Design review of the part built by this model. Coordinates are the model's own, in mm. Coordinates: 2 decimals unless noted, no trailing zeros. Write each loop counter-clockwise with the first axis right and the second up, starting at its lowest first coordinate (ties: lowest second). Pieces come first, ordered by that corner, then holes.
Q1. Clearance check with a flat-ended pin moving along its axis: pin 1 Ø5 at (x, y) = (-40.5, -4.5) entering from -Z. State where the tip first meets the part, or that it passes through.
Q2. Add section D-D, the plane y = -43. Give the boundary of the cut face in (x, z).
Q3. To check wall thickness, follow probe 1 along Y at (x, z) = (0, 0.85); probe 2 along Y at (x, z) = (17.5, 1.75); probe 3 along X at (y, z) = (0, 1.35). State the ranges of each line that lie inside material, in increasing order.
Q4. Add section C-C, the plane x = 0. Give the boundary of the cut face in (y, z).
Q5. Add section B-B, the plane z = 2.1. Give the boundary of the cut face in (x, y).
Q6. Add section A-A, the plane y = -14. Give the boundary of the cut face in (x, z).
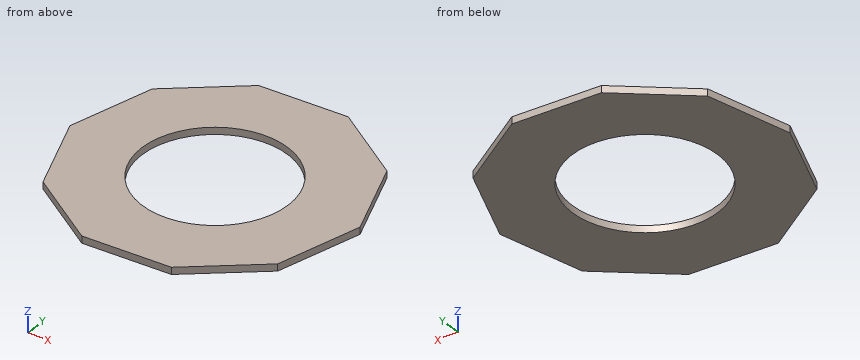
from build123d import *

# Parameters (mm, degrees)
F3_DEPTH = 2.54
F4_R     = 26.6451921389
F5_DEPTH = 25.4


# Not quite as in the source:
# - the program builds the solid bodies; features that only make, move or delete a surface that nothing else refers to are left out


with BuildPart() as f3:
    # F0 (on Top) → F3 (new body)
    with BuildSketch(Plane.XY):
        Polygon((13.1522906624, 49.1708465148), (-18.2614717633, 47.5107729435), (-42.69997266, 27.7031989396), (-50.8285353193, -2.6860554622), (-39.542325085, -32.049327973), (-13.1522906624, -49.1708465148), (18.2614717633, -47.5107729435), (42.69997266, -27.7031989396), (50.8285353193, 2.6860554622), (39.542325085, 32.049327973), align=None)
    extrude(amount=F3_DEPTH)

    # F4 (on face) → F5 (cut)
    with BuildSketch(Plane(origin=(0, 0, 0), x_dir=(1, 0, 0), z_dir=(0, 0, -1))):
        Circle(F4_R)
    extrude(amount=-F5_DEPTH, mode=Mode.SUBTRACT)


solid = f3.part
Here are the results:
1. pin 1: stops at z = 0
2. outline: (-22.66, 0) - (23.83, 0) - (23.83, 2.54) - (-22.66, 2.54) - close
3. probe 1: y = -48.48 to -26.65, 26.65 to 48.48
3. probe 2: y = -47.55 to -20.09, 20.09 to 46.35
3. probe 3: x = -50.11 to -26.65, 26.65 to 50.11
4. outline: (-48.48, 0) - (-26.65, 0) - (-26.65, 2.54) - (-48.48, 2.54) - close; (26.65, 0) - (48.48, 0) - (48.48, 2.54) - (26.65, 2.54) - close
5. outline: (-50.83, -2.69) - (-39.54, -32.05) - (-13.15, -49.17) - (18.26, -47.51) - (42.7, -27.7) - (50.83, 2.69) - (39.54, 32.05) - (13.15, 49.17) - (-18.26, 47.51) - (-42.7, 27.7) - close; hole circle Ø53.29 at (0, 0)
6. outline: (-46.48, 0) - (-22.67, 0) - (-22.67, 2.54) - (-46.48, 2.54) - close; (22.67, 0) - (46.37, 0) - (46.37, 2.54) - (22.67, 2.54) - close
